Input: part model. Units: mm. Frame: model coordinates. Face numbers are marked on the shaded views. A direction names the side the tool comes from. Give positions to 0.01 mm unless a question says otherwise; leave off trailing zeros. Order: outer loops, then holes, each group sorted by start corner. A loop starts at its lowest first (then second) coordinate and runs counter-clockwise, first axis right, second up. Notation, with made-up numbers: (74.5, 28) - (81.5, 28) arc R8 ccw to (81.5, 43) - close; hole circle Ø8 at (48.5, 23.25). An arc over 180 degrees is marked (long way). Use a Markdown table: item, result.
from build123d import *

# Parameters (mm, degrees)
CROQUIS1_R                   = 1.5
SALIENTE_EXTRUIR1_DEPTH      = 1.6
CROQUIS2_W                   = 4.4
CROQUIS2_H                   = 2.4
CROQUIS2_R                   = 0.1
CROQUIS2_R_2                 = 0.2
SALIENTE_EXTRUIR2_DEPTH      = 1
REDONDEO1_R                  = 1
SALIENTE_EXTRUIR3_DEPTH      = 2.54
SALIENTE_EXTRUIR4_DEPTH      = 6
SALIENTE_EXTRUIR4_DEPTH_BACK = 5


with BuildPart() as part:
    # Croquis1 → Saliente-Extruir1 (new body)
    with BuildSketch(Plane.XY):
        with BuildLine():
            Line((-8, -5.5), (8, -5.5))
            Line((8, -5.5), (8, -2.5))
            Line((8, -2.5), (10, -2.5))
            ThreePointArc((10, -2.5), (12.5, 0), (10, 2.5))
            Line((10, 2.5), (8, 2.5))
            Line((8, 2.5), (8, 5.5))
            Line((8, 5.5), (-8, 5.5))
            Line((-8, 5.5), (-8, 2.5))
            Line((-8, 2.5), (-10, 2.5))
            ThreePointArc((-10, 2.5), (-12.5, 0), (-10, -2.5))
            Line((-10, -2.5), (-8, -2.5))
            Line((-8, -2.5), (-8, -5.5))
        make_face()
        with Locations((10, 0)):
            Circle(CROQUIS1_R, mode=Mode.SUBTRACT)
        with Locations(Location((-10, 0, 0), (0, 0, 180))):
            Circle(CROQUIS1_R, mode=Mode.SUBTRACT)
    extrude(amount=SALIENTE_EXTRUIR1_DEPTH)

    # Croquis2 → Saliente-Extruir2 (add)
    with BuildSketch(Plane.XY.offset(1.6)):
        with Locations((0, -2.3)):
            Rectangle(CROQUIS2_W, CROQUIS2_H)
        with Locations((-1.535, -2.3)):
            Circle(CROQUIS2_R, mode=Mode.SUBTRACT)
        with Locations((1.465, -2.3)):
            Circle(CROQUIS2_R_2, mode=Mode.SUBTRACT)
    extrude(amount=SALIENTE_EXTRUIR2_DEPTH)

    # Redondeo1
    redondeo1_edges = [part.edges().sort_by_distance(p)[0] for p in [
        (8, 2.5, 0.8),
        (8, -2.5, 0.8),
        (-8, -2.5, 0.8),
        (-8, 2.5, 0.8),
    ]]
    fillet(redondeo1_edges, radius=REDONDEO1_R)

    # Croquis3 → Saliente-Extruir3 (add)
    with BuildSketch(Plane(origin=(0, 0, 0), x_dir=(-1, 0, 0), z_dir=(0, 0, -1))):
        with BuildLine():
            Line((0.3, 2.46), (2.24, 2.46))
            ThreePointArc((2.24, 2.46), (2.452132034, 2.547867966), (2.54, 2.76))
            ThreePointArc((2.54, 2.76), (2.627867966, 2.547867966), (2.84, 2.46))
            Line((2.84, 2.46), (4.78, 2.46))
            ThreePointArc((4.78, 2.46), (4.992132034, 2.547867966), (5.08, 2.76))
            ThreePointArc((5.08, 2.76), (5.167867966, 2.547867966), (5.38, 2.46))
            Line((5.38, 2.46), (7.32, 2.46))
            ThreePointArc((7.32, 2.46), (7.532132034, 2.547867966), (7.62, 2.76))
            Line((7.62, 2.76), (7.62, 4.7))
            ThreePointArc((7.62, 4.7), (7.532132034, 4.912132034), (7.32, 5))
            Line((7.32, 5), (5.38, 5))
            ThreePointArc((5.38, 5), (5.167867966, 4.912132034), (5.08, 4.7))
            ThreePointArc((5.08, 4.7), (4.992132034, 4.912132034), (4.78, 5))
            Line((4.78, 5), (2.84, 5))
            ThreePointArc((2.84, 5), (2.627867966, 4.912132034), (2.54, 4.7))
            ThreePointArc((2.54, 4.7), (2.452132034, 4.912132034), (2.24, 5))
            Line((2.24, 5), (0.3, 5))
            ThreePointArc((0.3, 5), (0.087867966, 4.912132034), (0, 4.7))
            ThreePointArc((0, 4.7), (-0.087867966, 4.912132034), (-0.3, 5))
            Line((-0.3, 5), (-2.24, 5))
            ThreePointArc((-2.24, 5), (-2.452132034, 4.912132034), (-2.54, 4.7))
            ThreePointArc((-2.54, 4.7), (-2.627867966, 4.912132034), (-2.84, 5))
            Line((-2.84, 5), (-4.78, 5))
            ThreePointArc((-4.78, 5), (-4.992132034, 4.912132034), (-5.08, 4.7))
            ThreePointArc((-5.08, 4.7), (-5.167867966, 4.912132034), (-5.38, 5))
            Line((-5.38, 5), (-7.32, 5))
            ThreePointArc((-7.32, 5), (-7.532132034, 4.912132034), (-7.62, 4.7))
            Line((-7.62, 4.7), (-7.62, 2.76))
            ThreePointArc((-7.62, 2.76), (-7.532132034, 2.547867966), (-7.32, 2.46))
            Line((-7.32, 2.46), (-5.38, 2.46))
            ThreePointArc((-5.38, 2.46), (-5.167867966, 2.547867966), (-5.08, 2.76))
            ThreePointArc((-5.08, 2.76), (-4.992132034, 2.547867966), (-4.78, 2.46))
            Line((-4.78, 2.46), (-2.84, 2.46))
            ThreePointArc((-2.84, 2.46), (-2.627867966, 2.547867966), (-2.54, 2.76))
            ThreePointArc((-2.54, 2.76), (-2.452132034, 2.547867966), (-2.24, 2.46))
            Line((-2.24, 2.46), (-0.3, 2.46))
            ThreePointArc((-0.3, 2.46), (-0.087867966, 2.547867966), (0, 2.76))
            ThreePointArc((0, 2.76), (0.087867966, 2.547867966), (0.3, 2.46))
        make_face()
    extrude(amount=SALIENTE_EXTRUIR3_DEPTH)

    # Croquis4 → Saliente-Extruir4 (add, two sides: drawn at the far end of the back side and taken through both)
    with BuildSketch(Plane(origin=(0, 0, -2.54), x_dir=(-1, 0, 0), z_dir=(0, 0, -1)).offset(-SALIENTE_EXTRUIR4_DEPTH_BACK)):
        Polygon((6.025, 3.505), (6.025, 3.955), (6.125, 4.055), (6.575, 4.055), (6.675, 3.955), (6.675, 3.505), (6.575, 3.405), (6.125, 3.405), align=None)
        Polygon((3.485, 3.505), (3.485, 3.955), (3.585, 4.055), (4.035, 4.055), (4.135, 3.955), (4.135, 3.505), (4.035, 3.405), (3.585, 3.405), align=None)
        Polygon((0.945, 3.505), (0.945, 3.955), (1.045, 4.055), (1.495, 4.055), (1.595, 3.955), (1.595, 3.505), (1.495, 3.405), (1.045, 3.405), align=None)
        Polygon((-4.135, 3.505), (-4.135, 3.955), (-4.035, 4.055), (-3.585, 4.055), (-3.485, 3.955), (-3.485, 3.505), (-3.585, 3.405), (-4.035, 3.405), align=None)
        Polygon((-1.595, 3.505), (-1.595, 3.955), (-1.495, 4.055), (-1.045, 4.055), (-0.945, 3.955), (-0.945, 3.505), (-1.045, 3.405), (-1.495, 3.405), align=None)
        Polygon((-6.675, 3.505), (-6.675, 3.955), (-6.575, 4.055), (-6.125, 4.055), (-6.025, 3.955), (-6.025, 3.505), (-6.125, 3.405), (-6.575, 3.405), align=None)
    extrude(amount=SALIENTE_EXTRUIR4_DEPTH + SALIENTE_EXTRUIR4_DEPTH_BACK)


solid = part.part
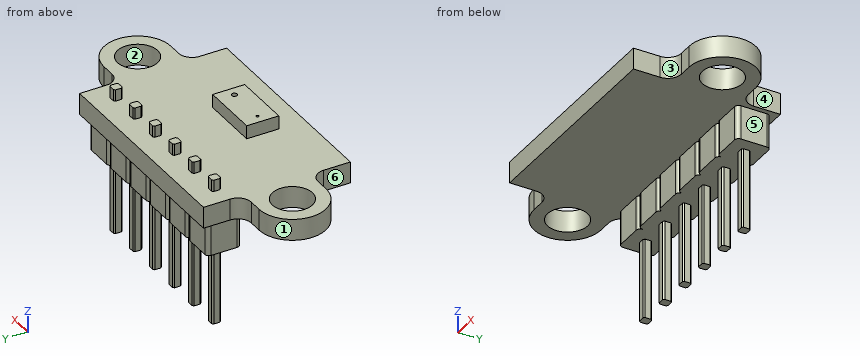
1. Pin query (flat end, axial travel): pin 1 (1.1 mm diameter, centred on x = 9.5, z = 0.5, fed in from +Y); pin 2 (1.1 mm diameter, centred on x = -0.5, z = 2, fed in from +Y); pin 3 (2 mm diameter, centred on x = 9.5, y = 1.5, fed in from -Z); pin 4 (2 mm diameter, centred on x = -3.5, z = -1.5, fed in from +Y). Return the tip coordinate at first contact, or that it passes through.
Response:
| item | result |
|---|---|
| pin 1 | stops at y = 2.5 |
| pin 2 | stops at y = 5.5 |
| pin 3 | stops at z = 0 |
| pin 4 | stops at y = 5 |
2. Section query C-C (y = 0). Return loops of the section in (x, z).
Response:
| item | result |
|---|---|
| outline | (-12.5, 0) - (-11.5, 0) - (-11.5, 1.6) - (-12.5, 1.6) - close; (-8.5, 0) - (8.5, 0) - (8.5, 1.6) - (-8.5, 1.6) - close; (11.5, 0) - (12.5, 0) - (12.5, 1.6) - (11.5, 1.6) - close |
3. Material intervals for line 1 along Y through (x, z) = (-6.5, -4.5) (3 decimals); line 2 along Z through (x, y) = (4.5, -5); line 3 along Y through (x, z) = (4.5, -0.75), sorted ascending.
Response:
| item | result |
|---|---|
| line 1 | y = 3.405 to 4.055 |
| line 2 | z = 0 to 1.6 |
| line 3 | y = 2.46 to 5 |
4. Section query A-A (z = 0.25). Return loops of the section in (x, y), then the cut area to 3 significant figures.
Response:
| item | result |
|---|---|
| outline | (-10, -2.5) - (-9, -2.5) arc R1 cw to (-8, -3.5) - (-8, -5.5) - (8, -5.5) - (8, -3.5) arc R1 cw to (9, -2.5) - (10, -2.5) arc R2.5 ccw to (10, 2.5) - (9, 2.5) arc R1 cw to (8, 3.5) - (8, 5.5) - (-8, 5.5) - (-8, 3.5) arc R1 cw to (-9, 2.5) - (-10, 2.5) arc R2.5 ccw to start; hole circle Ø3 at (-10, 0); hole circle Ø3 at (10, 0) |
| area | 202 mm^2 |
5. Section query D-D (y = -4.5). Return loops of the section in (x, z).
Response:
| item | result |
|---|---|
| outline | (-8, 0) - (8, 0) - (8, 1.6) - (-8, 1.6) - close |
6. Section query B-B (x = -4.5). Return loops of the section in (y, z).
Response:
| item | result |
|---|---|
| outline | (-5.5, 0) - (2.46, 0) - (2.46, -2.54) - (5, -2.54) - (5, 0) - (5.5, 0) - (5.5, 1.6) - (-5.5, 1.6) - close |
7. Set-up query: the marked faces 4, 5 and 6. Return all of +Z, -Z, +X, -X, +Y, -Y with unobstructed straight access to the full face (end or side cutting, diameter ignored); none if empty.
Response:
| item | result |
|---|---|
| face 4 | +Z, -Z, +X, +Y |
| face 5 | -Z, +X, +Y, -Y |
| face 6 | +Z, -Z, -X, -Y |
8. Mould query, pull axis Y, two halves, no side actions, for the marked faces 1, 2 and 3. Classes: pulls with the +Y half, pulls with the -Y half, needs draft (parallel to the pull), parting line crosses it, or undercut.
Response:
| item | result |
|---|---|
| face 1 | parting line crosses it |
| face 2 | undercut |
| face 3 | pulls with the -Y half |
